from build123d import *

# Parameters (mm, degrees)
SKETCH_1_W      = 84
SKETCH_1_H      = 44
EXTRUDE_1_DEPTH = 10
SKETCH_3_W      = 24.5
SKETCH_3_H      = 16.3
EXTRUDE_2_DEPTH = 2
FILLET_1_R      = 0.5
FILLET_2_R      = 0.5
FILLET_3_R      = 0.5


with BuildPart() as part:
    # 草图1 → 凸台-拉伸1 (new body)
    with BuildSketch(Plane(origin=(0, 0, 0), x_dir=(1, 0, 0), z_dir=(0, 1, 0))):
        Rectangle(SKETCH_1_W, SKETCH_1_H)
    extrude(amount=EXTRUDE_1_DEPTH)

    # 草图3 → 凸台-拉伸2 (add)
    with BuildSketch(Plane(origin=(0, 10, 0), x_dir=(1, 0, 0), z_dir=(0, 1, 0))):
        with Locations((-29.75, 0)):
            Rectangle(SKETCH_3_W, SKETCH_3_H)
    extrude(amount=EXTRUDE_2_DEPTH)

    # 圆角1
    fillet_1_edges = [part.edges().sort_by_distance(p)[0] for p in [
        (42, 10, 0),
    ]]
    fillet(fillet_1_edges, radius=FILLET_1_R)

    # 圆角2
    fillet_2_edges = [part.edges().sort_by_distance(p)[0] for p in [
        (-0.25, 10, 22),
        (42, 4.75, 22),
        (41.853553391, 9.853553391, 22),
        (0, 0, 22),
    ]]
    fillet(fillet_2_edges, radius=FILLET_2_R)

    # 圆角3
    # the kernel refuses this fillet: 0.5 mm, written as the material it takes off along each edge
    with BuildSketch(Plane(origin=(41.5, 0.5, 21.5), x_dir=(0, -1, 0), z_dir=(1, 0, 0))) as fillet_3_piece_1_section:
        Polygon((0, 0), (FILLET_3_R, 0), (FILLET_3_R, -FILLET_3_R), (0, -FILLET_3_R), align=None)
    fillet_3_piece_1 = extrude(amount=FILLET_3_R, mode=Mode.PRIVATE)
    fillet_3_piece_1 = fillet_3_piece_1 - Plane(origin=(41.5, 0.5, 21.5), x_dir=(0, 0.7071067811865475, -0.7071067811865475), z_dir=(1, 0, 0)) * Sphere(FILLET_3_R, mode=Mode.PRIVATE)
    add(fillet_3_piece_1, mode=Mode.SUBTRACT)
    with BuildSketch(Plane(origin=(41.5, 0.5, -21.5), x_dir=(0, 0, -1), z_dir=(1, 0, 0))) as fillet_3_piece_2_section:
        Polygon((0, 0), (FILLET_3_R, 0), (FILLET_3_R, -FILLET_3_R), (0, -FILLET_3_R), align=None)
    fillet_3_piece_2 = extrude(amount=FILLET_3_R, mode=Mode.PRIVATE)
    fillet_3_piece_2 = fillet_3_piece_2 - Plane(origin=(41.5, 0.5, -21.5), x_dir=(0, 0.7071067811865475, 0.7071067811865475), z_dir=(1, 0, 0)) * Sphere(FILLET_3_R, mode=Mode.PRIVATE)
    add(fillet_3_piece_2, mode=Mode.SUBTRACT)
    with BuildSketch(Plane(origin=(-41.5, 0.5, -21.5), x_dir=(0, 0, -1), z_dir=(-1, 0, 0))) as fillet_3_piece_3_section:
        Polygon((0, 0), (FILLET_3_R, 0), (FILLET_3_R, FILLET_3_R), (0, FILLET_3_R), align=None)
    fillet_3_piece_3 = extrude(amount=FILLET_3_R, mode=Mode.PRIVATE)
    fillet_3_piece_3 = fillet_3_piece_3 - Plane(origin=(-41.5, 0.5, -21.5), x_dir=(0, 0.7071067811865475, 0.7071067811865475), z_dir=(-1, 0, 0)) * Sphere(FILLET_3_R, mode=Mode.PRIVATE)
    add(fillet_3_piece_3, mode=Mode.SUBTRACT)
    with BuildSketch(Plane(origin=(-42, 10, 21.5), x_dir=(1, 0, 0), z_dir=(0, 0, -1))) as fillet_3_piece_4:
        with BuildLine():
            CenterArc((FILLET_3_R, FILLET_3_R), FILLET_3_R, 180, 90)
            Line((0, FILLET_3_R), (0, 0))
            Line((0, 0), (FILLET_3_R, 0))
        make_face()
    extrude(amount=13.35, mode=Mode.SUBTRACT)
    with BuildSketch(Plane(origin=(-42, 10, 8.15), x_dir=(0, 0, -1), z_dir=(0, 1, 0))) as fillet_3_piece_5:
        with BuildLine():
            CenterArc((FILLET_3_R, -FILLET_3_R), FILLET_3_R, 90, 90)
            Line((0, -FILLET_3_R), (0, 0))
            Line((0, 0), (FILLET_3_R, 0))
        make_face()
    extrude(amount=3.25, mode=Mode.SUBTRACT)
    with BuildSketch(Plane(origin=(-17.5, 10, -8.15), x_dir=(-1, 0, 0), z_dir=(0, 1, 0))) as fillet_3_piece_6:
        with BuildLine():
            CenterArc((FILLET_3_R, FILLET_3_R), FILLET_3_R, 180, 90)
            Line((0, FILLET_3_R), (0, 0))
            Line((0, 0), (FILLET_3_R, 0))
        make_face()
    extrude(amount=3.25, mode=Mode.SUBTRACT)
    with BuildSketch(Plane(origin=(-42, 12, -9.4), x_dir=(0, -1, 0), z_dir=(0, 0, 1))) as fillet_3_piece_7:
        with BuildLine():
            CenterArc((FILLET_3_R, FILLET_3_R), FILLET_3_R, 180, 90)
            Line((0, FILLET_3_R), (0, 0))
            Line((0, 0), (FILLET_3_R, 0))
        make_face()
    extrude(amount=18.8, mode=Mode.SUBTRACT)
    with BuildSketch(Plane(origin=(-16.25, 12, -8.15), x_dir=(0, -1, 0), z_dir=(-1, 0, 0))) as fillet_3_piece_8:
        with BuildLine():
            CenterArc((FILLET_3_R, FILLET_3_R), FILLET_3_R, 180, 90)
            Line((0, FILLET_3_R), (0, 0))
            Line((0, 0), (FILLET_3_R, 0))
        make_face()
    extrude(amount=27, mode=Mode.SUBTRACT)
    with BuildSketch(Plane(origin=(-43.25, 10, -22), x_dir=(0, -1, 0), z_dir=(1, 0, 0))) as fillet_3_piece_9:
        with BuildLine():
            CenterArc((FILLET_3_R, -FILLET_3_R), FILLET_3_R, 90, 90)
            Line((0, -FILLET_3_R), (0, 0))
            Line((0, 0), (FILLET_3_R, 0))
        make_face()
    extrude(amount=84.75, mode=Mode.SUBTRACT)
    with BuildSketch(Plane(origin=(42, 0.5, -22), x_dir=(0, 0, 1), z_dir=(0, 1, 0))) as fillet_3_piece_10:
        with BuildLine():
            CenterArc((FILLET_3_R, -FILLET_3_R), FILLET_3_R, 90, 90)
            Line((0, -FILLET_3_R), (0, 0))
            Line((0, 0), (FILLET_3_R, 0))
        make_face()
    extrude(amount=9, mode=Mode.SUBTRACT)
    with BuildSketch(Plane(origin=(41.5, 9.5, -22), x_dir=(1, 0, 0), z_dir=(0, -1, 0))) as fillet_3_piece_11:
        with BuildLine():
            CenterArc((0.5 - FILLET_3_R, FILLET_3_R), FILLET_3_R, 270, 90)
            Line((0.5 - FILLET_3_R, 0), (0.5, 0))
            Line((0.5, 0), (0.5, FILLET_3_R))
        make_face()
    revolve(axis=Axis((41.5, 9.5, -22), (0, 0, 1)), revolution_arc=90, mode=Mode.SUBTRACT)
    with BuildSketch(Plane(origin=(42, 0, -21.5), x_dir=(0, 1, 0), z_dir=(0, 0, 1))) as fillet_3_piece_12:
        with BuildLine():
            CenterArc((FILLET_3_R, FILLET_3_R), FILLET_3_R, 180, 90)
            Line((0, FILLET_3_R), (0, 0))
            Line((0, 0), (FILLET_3_R, 0))
        make_face()
    extrude(amount=43, mode=Mode.SUBTRACT)
    with BuildSketch(Plane(origin=(-42, 0.5, 22), x_dir=(1, 0, 0), z_dir=(0, 1, 0))) as fillet_3_piece_13:
        with BuildLine():
            CenterArc((FILLET_3_R, FILLET_3_R), FILLET_3_R, 180, 90)
            Line((0, FILLET_3_R), (0, 0))
            Line((0, 0), (FILLET_3_R, 0))
        make_face()
    extrude(amount=9, mode=Mode.SUBTRACT)
    with BuildSketch(Plane(origin=(-42, 0.5, 21.5), x_dir=(0, -1, 0), z_dir=(0, 0, -1))) as fillet_3_piece_14:
        with BuildLine():
            CenterArc((0.5 - FILLET_3_R, -FILLET_3_R), FILLET_3_R, 0, 90)
            Line((0.5 - FILLET_3_R, 0), (0.5, 0))
            Line((0.5, 0), (0.5, -FILLET_3_R))
        make_face()
    revolve(axis=Axis((-42, 0.5, 21.5), (-1, 0, 0)), revolution_arc=90, mode=Mode.SUBTRACT)
    with BuildSketch(Plane(origin=(-42, 9.5, 21.5), x_dir=(0, 1, 0), z_dir=(0, 0, -1))) as fillet_3_piece_15:
        with BuildLine():
            CenterArc((0.5 - FILLET_3_R, FILLET_3_R), FILLET_3_R, 270, 90)
            Line((0.5, FILLET_3_R), (0.5, 0))
            Line((0.5, 0), (0.5 - FILLET_3_R, 0))
        make_face()
    revolve(axis=Axis((-42, 9.5, 21.5), (1, 0, 0)), revolution_arc=90, mode=Mode.SUBTRACT)
    with BuildSketch(Plane(origin=(-42, 0, 21.5), x_dir=(1, 0, 0), z_dir=(0, 0, -1))) as fillet_3_piece_16:
        with BuildLine():
            CenterArc((FILLET_3_R, -FILLET_3_R), FILLET_3_R, 90, 90)
            Line((0, -FILLET_3_R), (0, 0))
            Line((0, 0), (FILLET_3_R, 0))
        make_face()
    extrude(amount=43, mode=Mode.SUBTRACT)
    with BuildSketch(Plane(origin=(-41.5, 0, -22), x_dir=(0, 1, 0), z_dir=(1, 0, 0))) as fillet_3_piece_17:
        with BuildLine():
            CenterArc((FILLET_3_R, FILLET_3_R), FILLET_3_R, 180, 90)
            Line((0, FILLET_3_R), (0, 0))
            Line((0, 0), (FILLET_3_R, 0))
        make_face()
    extrude(amount=83, mode=Mode.SUBTRACT)
    with BuildSketch(Plane(origin=(-42, 0.5, -22), x_dir=(1, 0, 0), z_dir=(0, 1, 0))) as fillet_3_piece_18:
        with BuildLine():
            CenterArc((FILLET_3_R, -FILLET_3_R), FILLET_3_R, 90, 90)
            Line((0, -FILLET_3_R), (0, 0))
            Line((0, 0), (FILLET_3_R, 0))
        make_face()
    extrude(amount=10.75, mode=Mode.SUBTRACT)
    with BuildSketch(Plane(origin=(-42, 10, 21.5), x_dir=(1, 0, 0), z_dir=(0, 0, -1))) as fillet_3_piece_19a_section:
        with BuildLine():
            CenterArc((FILLET_3_R, FILLET_3_R), FILLET_3_R, 180, 90)
            Line((0, FILLET_3_R), (0, 0))
            Line((0, 0), (FILLET_3_R, 0))
        make_face()
    fillet_3_piece_19a = extrude(amount=14.6, mode=Mode.PRIVATE)
    fillet_3_piece_19a = split(fillet_3_piece_19a, bisect_by=Plane(origin=(-41.886802443, 9.886802443, 8.15), z_dir=(0, 0, -1)), keep=Keep.TOP, mode=Mode.PRIVATE)
    with BuildSketch(Plane(origin=(-42, 8.75, 8.15), x_dir=(0, 0, -1), z_dir=(0, 1, 0))) as fillet_3_piece_19b_section:
        with BuildLine():
            CenterArc((FILLET_3_R, -FILLET_3_R), FILLET_3_R, 90, 90)
            Line((0, -FILLET_3_R), (0, 0))
            Line((0, 0), (FILLET_3_R, 0))
        make_face()
    fillet_3_piece_19b = extrude(amount=4.5, mode=Mode.PRIVATE)
    fillet_3_piece_19b = split(fillet_3_piece_19b, bisect_by=Plane(origin=(-41.886802443, 10, 8.036802443), z_dir=(0, -1, 0)), keep=Keep.TOP, mode=Mode.PRIVATE)
    fillet_3_piece_19 = fillet_3_piece_19a & fillet_3_piece_19b
    add(fillet_3_piece_19, mode=Mode.SUBTRACT)
    # the kernel refuses this fillet: 0.5 mm, written as the material it adds along each edge
    with BuildSketch(Plane(origin=(-17.5, 10, 8.15), x_dir=(0, 1, 0), z_dir=(0, 0, -1))) as fillet_3_2_piece_1:
        with BuildLine():
            CenterArc((FILLET_3_R, FILLET_3_R), FILLET_3_R, 180, 90)
            Line((0, FILLET_3_R), (0, 0))
            Line((0, 0), (FILLET_3_R, 0))
        make_face()
    extrude(amount=15.8)
    with BuildSketch(Plane(origin=(-18, 10, -8.15), x_dir=(0, 1, 0), z_dir=(-1, 0, 0))) as fillet_3_2_piece_2:
        with BuildLine():
            CenterArc((FILLET_3_R, FILLET_3_R), FILLET_3_R, 180, 90)
            Line((0, FILLET_3_R), (0, 0))
            Line((0, 0), (FILLET_3_R, 0))
        make_face()
    extrude(amount=24)
    with BuildSketch(Plane(origin=(-18, 10, -7.65), x_dir=(0, 0, -1), z_dir=(-1, 0, 0))) as fillet_3_2_piece_3:
        with BuildLine():
            CenterArc((0.5 + FILLET_3_R, -FILLET_3_R), FILLET_3_R, 90, 90)
            Line((0.5 + FILLET_3_R, 0), (0.5, 0))
            Line((0.5, 0), (0.5, -FILLET_3_R))
        make_face()
    revolve(axis=Axis((-18, 10, -7.65), (0, -1, 0)), revolution_arc=90)
    # the kernel refuses this fillet: 0.5 mm, written as the material it takes off along each edge
    with BuildSketch(Plane(origin=(-41.5, 11.5, -7.65), x_dir=(-1, 0, 0), z_dir=(0, 0, -1))) as fillet_3_3_piece_1_section:
        Polygon((0, 0), (FILLET_3_R, 0), (FILLET_3_R, FILLET_3_R), (0, FILLET_3_R), align=None)
    fillet_3_3_piece_1 = extrude(amount=FILLET_3_R, mode=Mode.PRIVATE)
    fillet_3_3_piece_1 = fillet_3_3_piece_1 - Plane(origin=(-41.5, 11.5, -7.65), x_dir=(0.7071067811865475, -0.7071067811865475, 0), z_dir=(0, 0, -1)) * Sphere(FILLET_3_R, mode=Mode.PRIVATE)
    add(fillet_3_3_piece_1, mode=Mode.SUBTRACT)
    with BuildSketch(Plane(origin=(-41.5, 9.5, -21.5), x_dir=(0, 1, 0), z_dir=(-1, 0, 0))) as fillet_3_3_piece_2_section:
        Polygon((0, 0), (FILLET_3_R, 0), (FILLET_3_R, FILLET_3_R), (0, FILLET_3_R), align=None)
    fillet_3_3_piece_2 = extrude(amount=FILLET_3_R, mode=Mode.PRIVATE)
    fillet_3_3_piece_2 = fillet_3_3_piece_2 - Plane(origin=(-41.5, 9.5, -21.5), x_dir=(0, -0.7071067811865475, 0.7071067811865475), z_dir=(-1, 0, 0)) * Sphere(FILLET_3_R, mode=Mode.PRIVATE)
    add(fillet_3_3_piece_2, mode=Mode.SUBTRACT)
    with BuildSketch(Plane(origin=(-42, 10, -8.65), x_dir=(0, -1, 0), z_dir=(0, 0, -1))) as fillet_3_3_piece_3:
        with BuildLine():
            CenterArc((FILLET_3_R, -FILLET_3_R), FILLET_3_R, 90, 90)
            Line((0, -FILLET_3_R), (0, 0))
            Line((0, 0), (FILLET_3_R, 0))
        make_face()
    extrude(amount=12.85, mode=Mode.SUBTRACT)
    with BuildSketch(Plane(origin=(-42, 10.5, -8.15), x_dir=(1, 0, 0), z_dir=(0, 1, 0))) as fillet_3_3_piece_4:
        with BuildLine():
            CenterArc((FILLET_3_R, -FILLET_3_R), FILLET_3_R, 90, 90)
            Line((0, -FILLET_3_R), (0, 0))
            Line((0, 0), (FILLET_3_R, 0))
        make_face()
    extrude(amount=1, mode=Mode.SUBTRACT)
    with BuildSketch(Plane(origin=(-42, 10.5, -8.65), x_dir=(0, 0, 1), z_dir=(0, 1, 0))) as fillet_3_3_piece_5:
        with BuildLine():
            CenterArc((0.5 + FILLET_3_R, FILLET_3_R), FILLET_3_R, 180, 90)
            Line((0.5 + FILLET_3_R, 0), (0.5, 0))
            Line((0.5, 0), (0.5, FILLET_3_R))
        make_face()
    revolve(axis=Axis((-42, 10.5, -8.65), (1, 0, 0)), revolution_arc=90, mode=Mode.SUBTRACT)


solid = part.part
Read the model definition and answer for the solid it produces. Units are mm, in the model's axes. A direction names the side the tool comes from. Give positions to 0.01 mm unless a question says otherwise; leave off trailing zeros. Write each loop counter-clockwise with the first axis right and the second up, starting at its lowest first coordinate (ties: lowest second). Pieces come first, ordered by that corner, then holes. Notation, with made-up numbers: (-29.5, 78) - (-9.5, 78) arc R14 cw to (-9.5, 82) - close; hole circle Ø10 at (40.25, -37.5). An arc over 180 degrees is marked (long way). Answer in a Markdown table with one row per item. Add a question column.
Item 1: Section B-B, the plane z = 15 is taken. Write down the section's boundary in (x, y), and give its area (3 significant figures).
Item 2: Section D-D, the plane z = -6 is taken. Write down the section's boundary in (x, y).
Item 3: Flat-ended cylindrical pins translate along their axes: P1, Ø13, axis at x = 9, z = -5, coming from the +Y side; P2, Ø1.2, axis at y = 11.5, z = 3.5, coming from the +X side; P3, Ø1.1, axis at x = -27.5, y = 11, coming from the -Z side; P4, Ø6, axis at x = -24.5, z = -11.5, coming from the -Y side. Find the tip coordinate at first contact, or state that the pin passes through.
Item 4: Section C-C, the plane x = -21 is taken. Write down the section's boundary in (y, z), and give its area (3 significant figures).
Item 5: Section A-A, the plane x = 14 is taken. Write down the section's boundary in (y, z).
Item 6: A tool of negligible diameter and unlimited length cuts with its end or side. For faces 1 (the face through (-17.5, 11, 0)), 2 (the face through (-29, 11, 8.15)), 3 (the face through (-1, 10, 0)), 4 (the face through (-1, 0, 0)), from which of +Z, -Z, +X, -X, +Y, -Y can it reach the whole face along a straight path? Write none if from no direction.
Item 7: Find the intervals of material crossed by L1, parallel to Y at x = 24.5, z = 15; L2, parallel to X at y = 11.5, z = -6; L3, parallel to Z at x = -32, y = 10.75, in increasing order.
Recorded:
| question | item | result |
|---|---|---|
| 1 | outline | (-42, 0.5) arc R0.5 ccw to (-41.5, 0) - (41.5, 0) arc R0.5 ccw to (42, 0.5) - (42, 9.5) arc R0.5 ccw to (41.5, 10) - (-41.5, 10) arc R0.5 ccw to (-42, 9.5) - close |
| 1 | area | 840 mm2 |
| 2 | outline | (-42, 0.5) arc R0.5 ccw to (-41.5, 0) - (41.5, 0) arc R0.5 ccw to (42, 0.5) - (42, 9.5) arc R0.5 ccw to (41.5, 10) - (-17, 10) arc R0.5 cw to (-17.5, 10.5) - (-17.5, 12) - (-41.5, 12) arc R0.5 ccw to (-42, 11.5) - close |
| 3 | P1 | stops at y = 10 |
| 3 | P2 | stops at x = -17.5 |
| 3 | P3 | stops at z = -8.15 |
| 3 | P4 | stops at y = 0 |
| 4 | outline | (0, -21.5) arc R0.5 ccw to (0.5, -22) - (9.5, -22) arc R0.5 ccw to (10, -21.5) - (10, -8.65) arc R0.5 cw to (10.5, -8.15) - (11.5, -8.15) arc R0.5 ccw to (12, -7.65) - (12, 8.15) - (10, 8.15) - (10, 21.5) arc R0.5 ccw to (9.5, 22) - (0.5, 22) arc R0.5 ccw to (0, 21.5) - close |
| 4 | area | 472 mm2 |
| 5 | outline | (0, -21.5) arc R0.5 ccw to (0.5, -22) - (9.5, -22) arc R0.5 ccw to (10, -21.5) - (10, 21.5) arc R0.5 ccw to (9.5, 22) - (0.5, 22) arc R0.5 ccw to (0, 21.5) - close |
| 6 | face 1 | +Z, -Z, +X, +Y |
| 6 | face 2 | +Z, +X, -X, +Y |
| 6 | face 3 | +X, +Y |
| 6 | face 4 | +Z, -Z, +X, -X, -Y |
| 7 | L1 | y = 0 to 10 |
| 7 | L2 | x = -42 to -17.5 |
| 7 | L3 | z = -8.15 to 8.15 |
